```python
from build123d import *

# Parameters (mm, degrees)
CUT_EXTRUDE1_REACH      = 142.114
CUT_EXTRUDE1_END_RADIUS = 19.05
SKETCH3_R               = 6.35
SKETCH6_R               = 6.35
BOSS_EXTRUDE1_DEPTH     = 304.8


with BuildPart() as part:
    # Sketch1 → Revolve1 (revolve)
    with BuildSketch(Plane.XY, mode=Mode.PRIVATE) as revolve1_sk:
        with BuildLine():
            Line((-137.5, 0), (137.5, 0))
            Line((137.5, 0), (137.5, 7.747))
            add(Edge.make_bspline(
                [(119.602, 16.764), (126.446685513, 16.474787936), (132.251729161, 15.730759902), (137.5, 12.322795174), (137.5, 7.747)],
                knots=[0, 0, 0, 0, 0.656247862, 1, 1, 1, 1], degree=3))
            Line((119.602, 16.764), (65.5, 19.05))
            Line((65.5, 19.05), (-14.564, 19.05))
            add(Edge.make_bspline(
                [(-91.78, 17.399), (-84.901336541, 18.220618135), (-60.549292723, 10.012805319), (-35.82944709, 19.05), (-14.564, 19.05)],
                knots=[0, 0, 0, 0, 0.244238151, 1, 1, 1, 1], degree=3))
            Line((-91.78, 17.399), (-137.5, 11.938))
            Line((-137.5, 11.938), (-137.5, 0))
        make_face()
    revolve(revolve1_sk.sketch.rotate(Axis((-137.5, 0, 0), (1, 0, 0)), 180), axis=Axis((-137.5, 0, 0), (1, 0, 0)))

    # Cut-Extrude1: up to this cylinder (the profile starts inside it)
    cut_extrude1_end = Plane(origin=(12.36, 0, 0), z_dir=(-1, 0, 0)) * Cylinder(CUT_EXTRUDE1_END_RADIUS, 323.328, mode=Mode.PRIVATE)
    # Sketch3 → Cut-Extrude1 (cut, up to the surface)
    with BuildSketch(Plane(origin=(0, 0, 0), x_dir=(1, 0, 0), z_dir=(0, 1, 0)), mode=Mode.PRIVATE) as cut_extrude1_sk1:
        with Locations(Location((12.36, 0, 0), (0, 0, 90))):
            Circle(SKETCH3_R)
    cut_extrude1_tool1 = extrude(cut_extrude1_sk1.sketch, amount=CUT_EXTRUDE1_REACH, mode=Mode.PRIVATE) & cut_extrude1_end
    add(cut_extrude1_tool1.solids().sort_by_distance((12.36, 0, 0))[0], mode=Mode.SUBTRACT)

    # Sketch6 → Boss-Extrude1 (add)
    with BuildSketch(Plane.ZY.offset(137.5)):
        with Locations(Location((0, 0, 0), (0, 0, 90))):
            Circle(SKETCH6_R)
    extrude(amount=BOSS_EXTRUDE1_DEPTH)


solid = part.part
```
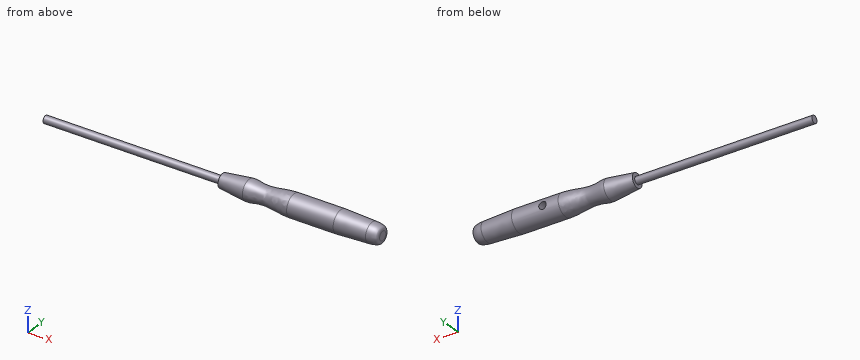
Source: CAD feature listing. Evaluate the final solid. Frame: model axes, mm. Round coordinates to 2 decimals unless told otherwise and drop trailing zeros. Loops run counter-clockwise (first coordinate to the right, second up) from the corner with the lowest first, then second, coordinate; pieces in that order, holes last.
1. Section query A-A on x = -331.5. Output: boundary loops of the cut face in (y, z), and give its area (3 significant figures).
2. Section query B-B on x = 12.36. Output: boundary loops of the cut face in (y, z), and give its area (3 significant figures).
3. Contact query for flat-ended pins moving along their axis: pin 1 (7.5 mm diameter, centred on x = 12.36, z = 0, fed in from +Y); pin 2 (6 mm diameter, centred on x = -195.5, y = 6.5, fed in from -Z); pin 3 (12 mm diameter, centred on x = -282.5, z = -5.5, fed in from -Y). Output: stop coordinate, or through.
4. Ray query, L1, parallel to X at y = 9.5, z = 0; L2, parallel to X at y = -5.5, z = 4; L3, parallel to X at y = 4.5, z = 0. Return the intervals inside material, ascending.
Answers below:
1. outline: circle Ø12.7 at (0, 0)
1. area: 127 mm2
2. outline: (0, -6.35) - (0, 6.35) - (17.96, 6.35) arc R19.05 ccw (long way) to (17.96, -6.35) - close
2. area: 903 mm2
3. pin 1: stops at y = 0
3. pin 2: stops at z = -5.3
3. pin 3: stops at y = -6.35
4. L1: x = -137.5 to 6.01, 18.71 to 137.4
4. L2: x = -137.5 to 137.5
4. L3: x = -442.3 to 6.01, 18.71 to 137.5
